Autodesk Inventor part; units mm, degrees
ref_plane "YZ Plane" through (0, 0, 0) normal (1, 0, 0) x (0, 1, 0)
ref_plane "XZ Plane" through (0, 0, 0) normal (0, 1, 0) x (-1, 0, 0)
ref_plane "XY Plane" through (0, 0, 0) normal (0, 0, 1) x (1, 0, 0)
sketch "Sketch1" plane through (0, 0, 0) normal (0, 1, 0) x (-1, 0, 0)
  line L0 (0, 0) -> (0, -521.938) construction
  line L1 (-4, 0) -> (-4, -521.938)
  line L2 (4, -521.938) -> (4, 0)
  arc A0 (4, 0) -> (-4, 0) centre (0, 0) ccw
  arc A1 (-4, -521.938) -> (4, -521.938) centre (0, -521.938) ccw
  circle A2 centre (0, 0) radius 1.5
  circle A3 centre (0, -521.938) radius 1.5
  arc A4 (-4, -3) -> (-4, -518.938) centre (537.7121, -260.969) ccw
  arc A5 (4, -3) -> (4, -518.938) centre (545.7121, -260.969) ccw
  point P0 (0, -260.969)
  point P1 (-4, -501.4199)
  point P2 (-4, -20.5181)
  dimension "d0" = 8
  dimension "d1" = 521.938
  dimension "d2" = 3
  dimension "d3" = 3
  dimension "d24" = 600
  dimension "d25" = 600
  dimension "d26" = 3
  dimension "d27" = 3
extrude "Extrusion1" add sketch "Sketch1" along normal blind 10 contours A0 L2 A5 L1 | L1 A5 A4 | L1 A5 L2 A1
sketch "Sketch5" plane through (0, 10, 0) normal (0, 1, 0) x (1, 0, 0)
  arc A0 (4, 3) -> (4, 518.938) centre (-537.7121, 260.969) ccw
  line L0 (4, 518.938) -> (4, 521.938)
  arc A1 (4, 521.938) -> (-4, 521.938) centre (0, 521.938) ccw
  line L1 (-4, 521.938) -> (-4, 518.938)
  arc A2 (-4, 3) -> (-4, 518.938) centre (-545.7121, 260.969) ccw
  line L2 (-4, 3) -> (-4, 0)
  arc A3 (-4, 0) -> (4, 0) centre (0, 0) ccw
  line L3 (4, 0) -> (4, 3)
  circle A4 centre (0, 521.938) radius 1.5
  circle A5 centre (0, 0) radius 1.5
  circle A6 centre (0, 521.938) radius 11
  point P0 (6.6919, 513.2076)
  point P1 (-0.2637, 510.9412)
  dimension "d45" = 22
extrude "Extrusion5" add sketch "Sketch5" against normal blind 10 contours A0 L0 A1 L1 A2 A6 picked at (6.2374, 520.1049)
sketch "Sketch6" plane through (0, 10, 0) normal (0, 1, 0) x (1, 0, 0)
  arc A0 (4, 3) -> (6.6919, 513.2076) centre (-537.7121, 260.969) ccw
  arc A1 (6.6919, 513.2076) -> (-0.2637, 510.9412) centre (0, 521.938) ccw
  arc A2 (-4, 3) -> (-0.2637, 510.9412) centre (-545.7121, 260.969) ccw
  line L0 (-4, 3) -> (-4, 0)
  arc A3 (-4, 0) -> (4, 0) centre (0, 0) ccw
  line L1 (4, 0) -> (4, 3)
  circle A4 centre (0, 521.938) radius 1.5
  circle A5 centre (0, 0) radius 1.5
  circle A6 centre (0, 529.938) radius 1.1
  circle A7 centre (0, 521.938) radius 4.25
  dimension "d48" = 2.2
  dimension "d49" = 8
  dimension "d55" = 8.5
extrude "Extrusion6" cut sketch "Sketch6" against normal blind 100 contours A4 | A6 | A7
pattern_circular "Circular Pattern1" count 8 over 360 about axis through (0, 0, -521.938) along (0, 1, 0) of "Extrusion6"
sketch "Sketch2" plane through (0, 10, 0) normal (0, 1, 0) x (1, 0, 0)
  arc A0 (4, 3) -> (6.6919, 513.2076) centre (-537.7121, 260.969) ccw
  arc A1 (-4, 3) -> (-0.2637, 510.9412) centre (-545.7121, 260.969) ccw
  line L0 (-4, 3) -> (-4, 0)
  arc A2 (-4, 0) -> (4, 0) centre (0, 0) ccw
  line L1 (4, 0) -> (4, 3)
  circle A3 centre (0, 0) radius 1.5
  arc A4 (-4, 3) -> (-4, 518.938) centre (-545.7121, 260.969) ccw
  line L2 (54.2879, 260.969) -> (58.1281, 268.7691)
  line L3 (58.1281, 268.7691) -> (62.2796, 257.8034)
  arc A5 (4, 3) -> (4, 518.938) centre (-537.7121, 260.969) ccw
  arc A6 (6.6919, 513.2076) -> (-0.2637, 510.9412) centre (0, 521.938) ccw
extrude "Extrusion2" [suppressed]
Can you work these out from the model? Positions are in its coordinate system, mm. Coordinates: 2 decimals unless noted, no trailing zeros. Loops run counter-clockwise (first coordinate to the right, second up) from the corner with the lowest first, then second, coordinate; pieces in that order, holes last. Notation, with made-up numbers: (40, 85.25) - (68, 85.25) arc R23 ccw to (68, 123.25) - close; hole circle Ø8 at (52.25, 60). An arc over 180 degrees is marked (long way). Use a Markdown table: item, result.
Item 1: If I drill on probe 1 along Z at (x, y) = (0, 3.25); probe 2 along X at (y, z) = (4.5, -105); probe 3 along X at (y, z) = (9.75, -71), over which ranges is the centre line in solid material (lowest first)? Write a range as from..to.
Numbers:
| item | result |
|---|---|
| probe 1 | z = -532.94..-531.04, -528.84..-526.19, -517.69..-515.04, -512.84..-510.36, -11.57..-1.5, 1.5..4 |
| probe 2 | x = 33.66..41.66 |
| probe 3 | x = 23.42..31.42 |
Item 2: Will these pins go through, and if not, where does the flat tip stop? pin 1 (5 mm diameter, centred on x = 2, y = 4.5, fed in from +Z); pin 2 (5 mm diameter, centred on x = 14, y = 3, fed in from +Z); pin 3 (1 mm diameter, centred on y = 1, z = -92, fed in from +X); pin 4 (0.9 mm diameter, centred on y = 4, z = -1, fed in from -X).
Numbers:
| item | result |
|---|---|
| pin 1 | stops at z = 4 |
| pin 2 | stops at z = -19.38 |
| pin 3 | stops at x = 38.15 |
| pin 4 | stops at x = -4 |
Item 3: I want a section at B-B on x = 41.5. Please give me the cut outline in (y, z), and give its area (3 significant figures).
Numbers:
| item | result |
|---|---|
| outline | (0, -417.54) - (10, -417.54) - (10, -384.18) - (0, -384.18) - close; (0, -137.75) - (10, -137.75) - (10, -104.4) - (0, -104.4) - close |
| area | 667 mm2 |
Item 4: I want a section at C-C on z = -358. Please give me the cut outline in (x, y), and give its area (3 significant figures).
Numbers:
| item | result |
|---|---|
| outline | (46.39, 0) - (54.39, 0) - (54.39, 10) - (46.39, 10) - close |
| area | 80.0 mm2 |
Item 5: I want a section at A-A on y = 3. Give the number of separate pieces and of enclosed holes in the cut face, and give its area (3 significant figures).
Numbers:
| item | result |
|---|---|
| separate pieces | 1 |
| enclosed holes | 10 |
| area | 4,400 mm2 |
Item 6: We'd pull the mould along X, two halves only. Please class faces 1 (the face through (62.288, 4.93, -261.492)), 2 (the face through (55, 0, -266)), 3 (the face through (-0.553, 5.07, -526.152)), 4 (the face through (-3, 5.07, -532.52)): released by +X, released by -X, zero draft, split by the parting line, or undercut.
Numbers:
| item | result |
|---|---|
| face 1 | released by +X |
| face 2 | zero draft |
| face 3 | undercut |
| face 4 | split by the parting line |
